```python
from build123d import *

# Parameters (mm, degrees)
SKETCH_1_W               = 50
SKETCH_1_H               = 50
EXTRUDE_1_DEPTH          = 10
SKETCH_2_R               = 1.75
EXTRUDE_2_DEPTH          = 2.25
CUT_EXTRUDE_1_DEPTH      = 71.505318948
CUT_EXTRUDE_1_DEPTH_BACK = 71.505318948
SKETCH_5_R               = 1.75
CUT_EXTRUDE_3_DEPTH      = 71.505318948
CUT_EXTRUDE_3_DEPTH_BACK = 5
SKETCH_6_R               = 3.3
FILLET_1_R               = 10
SKETCH_8_R               = 5.5
CUT_EXTRUDE_5_DEPTH      = 6.5
EXTRUDE_3_DEPTH          = 3
EXTRUDE_4_DEPTH          = 3
FILLET_2_R               = 1


with BuildPart() as part:
    # ｽｹｯﾁ1 → ﾎﾞｽ - 押し出し1 (new body)
    with BuildSketch(Plane(origin=(0, 0, 0), x_dir=(1, 0, 0), z_dir=(0, 1, 0))):
        Rectangle(SKETCH_1_W, SKETCH_1_H)
    extrude(amount=EXTRUDE_1_DEPTH)

    # ｽｹｯﾁ2 → ﾎﾞｽ - 押し出し2 (add, symmetric)
    with BuildSketch(Plane.XY):
        with BuildLine():
            Line((25, 10), (-25, 10))
            Line((-25, 10), (-25, 36))
            ThreePointArc((-25, 36), (0, 61), (25, 36))
            Line((25, 36), (25, 10))
        make_face()
        with Locations((0, 36)):
            Circle(SKETCH_2_R, mode=Mode.SUBTRACT)
    extrude(amount=EXTRUDE_2_DEPTH, both=True)

    # ｽｹｯﾁ5 → ｶｯﾄ - 押し出し1 (cut, two sides: drawn at the far end of the back side and taken through both)
    with BuildSketch(Plane.XY.offset(-CUT_EXTRUDE_1_DEPTH_BACK)):
        with Locations((0, 57)):
            Circle(SKETCH_5_R)
        with Locations((5.435199947, 56.284442352)):
            Circle(SKETCH_5_R)
        with Locations((10.5, 54.186533479)):
            Circle(SKETCH_5_R)
        with Locations((14.849242405, 50.849242405)):
            Circle(SKETCH_5_R)
        with Locations((18.186533479, 46.5)):
            Circle(SKETCH_5_R)
        with Locations((18.186533479, 25.5)):
            Circle(SKETCH_5_R)
        with Locations((14.849242405, 21.150757595)):
            Circle(SKETCH_5_R)
        with Locations((10.5, 17.813466521)):
            Circle(SKETCH_5_R)
        with Locations((5.435199947, 15.715557648)):
            Circle(SKETCH_5_R)
        with Locations((0, 15)):
            Circle(SKETCH_5_R)
        with Locations((-5.435199947, 15.715557648)):
            Circle(SKETCH_5_R)
        with Locations((-10.5, 17.813466521)):
            Circle(SKETCH_5_R)
        with Locations((-14.849242405, 21.150757595)):
            Circle(SKETCH_5_R)
        with Locations((-18.186533479, 25.5)):
            Circle(SKETCH_5_R)
        with Locations((-18.186533479, 46.5)):
            Circle(SKETCH_5_R)
        with Locations((-14.849242405, 50.849242405)):
            Circle(SKETCH_5_R)
        with Locations((-10.5, 54.186533479)):
            Circle(SKETCH_5_R)
        with Locations((-5.435199947, 56.284442352)):
            Circle(SKETCH_5_R)
    extrude(amount=CUT_EXTRUDE_1_DEPTH + CUT_EXTRUDE_1_DEPTH_BACK, mode=Mode.SUBTRACT)

    # ｽｹｯﾁ6 → ｶｯﾄ - 押し出し3 (cut, two sides: drawn at the far end of the back side and taken through both)
    with BuildSketch(Plane(origin=(0, 0, 0), x_dir=(1, 0, 0), z_dir=(0, 1, 0)).offset(-CUT_EXTRUDE_3_DEPTH_BACK)):
        with Locations(Location((-10, -10, 0), (0, 0, 90))):
            Circle(SKETCH_6_R)
        with Locations(Location((10, -10, 0), (0, 0, 90))):
            Circle(SKETCH_6_R)
        with Locations(Location((10, 10, 0), (0, 0, 90))):
            Circle(SKETCH_6_R)
        with Locations(Location((-10, 10, 0), (0, 0, 90))):
            Circle(SKETCH_6_R)
    extrude(amount=CUT_EXTRUDE_3_DEPTH + CUT_EXTRUDE_3_DEPTH_BACK, mode=Mode.SUBTRACT)

    # ﾌｨﾚｯﾄ1
    fillet_1_edges = [part.edges().sort_by_distance(p)[0] for p in [
        (-25, 5, 25),
        (-25, 5, -25),
        (25, 5, -25),
        (25, 5, 25),
    ]]
    fillet(fillet_1_edges, radius=FILLET_1_R)

    # ｽｹｯﾁ8 → ｶｯﾄ - 押し出し5 (cut)
    with BuildSketch(Plane(origin=(0, 10, 0), x_dir=(1, 0, 0), z_dir=(0, 1, 0))):
        with Locations(Location((-10, -10, 0), (0, 0, 270))):
            Circle(SKETCH_8_R)
        with Locations(Location((10, -10, 0), (0, 0, 270))):
            Circle(SKETCH_8_R)
        with Locations(Location((10, 10, 0), (0, 0, 270))):
            Circle(SKETCH_8_R)
        with Locations(Location((-10, 10, 0), (0, 0, 270))):
            Circle(SKETCH_8_R)
    extrude(amount=-CUT_EXTRUDE_5_DEPTH, mode=Mode.SUBTRACT)

    # ｽｹｯﾁ11 → ﾎﾞｽ - 押し出し3 (add)
    with BuildSketch(Plane(origin=(25, 0, 0), x_dir=(0, 0, -1), z_dir=(1, 0, 0))):
        Polygon((-2.25, 19.834192463), (-15, 10), (-2.25, 10), align=None)
        Polygon((15, 10), (2.25, 10), (2.25, 19.834192463), align=None)
    extrude(amount=-EXTRUDE_3_DEPTH)

    # ｽｹｯﾁ12 → ﾎﾞｽ - 押し出し4 (add)
    with BuildSketch(Plane.ZY.offset(25)):
        Polygon((2.25, 19.834192463), (15, 10), (2.25, 10), align=None)
        Polygon((-2.25, 19.834192463), (-15, 10), (-2.25, 10), align=None)
    extrude(amount=-EXTRUDE_4_DEPTH)

    # ﾌｨﾚｯﾄ2
    fillet_2_edges = [part.edges().sort_by_distance(p)[0] for p in [
        (0, 10, 2.25),
        (0, 10, -2.25),
    ]]
    fillet(fillet_2_edges, radius=FILLET_2_R)


solid = part.part
```
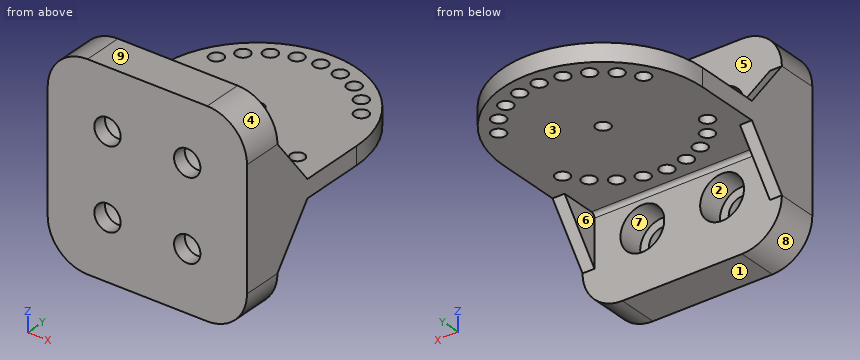
The model under review builds one solid part; all positions refer to its coordinate system, in mm. Face numbers are marked on the shaded views. A direction names the side the tool comes from. Give positions to 0.01 mm unless a question says otherwise; leave off trailing zeros. Write each loop counter-clockwise with the first axis right and the second up, starting at its lowest first coordinate (ties: lowest second). Pieces come first, ordered by that corner, then holes. Notation, with made-up numbers: (-31.5, 62) - (-0.5, 62) arc R16 ccw to (-0.5, 91) - close; hole circle Ø3 at (13, 36). An arc over 180 degrees is marked (long way). Answer in a Markdown table with one row per item. Add a question column.
1. Insertion check: P1, Ø4, axis at x = 10, z = -10, coming from the -Y side (3 decimals); P2, Ø5, axis at x = -18, y = 55, coming from the +Z side; P3, Ø4.5, axis at x = -5.44, y = 56.28, coming from the -Z side; P4, Ø4, axis at x = -18.5, z = -15, coming from the +Y side. Each pin has a flat end and moves straight along its axis. Give the tip position at first contact, or say it passes through.
2. Wall thickness on line 1 along X through (y, z) = (6.75, 10); line 2 along X through (y, z) = (7, -9); line 3 along Y through (x, z) = (3.5, 14): over which ranges is each line inside the solid? List them lowest first. Write a range as [from, to].
3. We need section B-B on y = 25.5. Write out the cut boundary in (x, z).
4. Draft analysis for pull direction Z (two halves, no side actions). For the marked faces 6, 7, 8 and 9, state which applies: +Z half, -Z half, draft (parallel to the pull), parting line (faces both ways), or undercut.
5. Tool access review of the marked faces 1, 2, 3, 4 and 5: name each direction out of +Z, -Z, +X, -X, +Y, -Y from which nothing blocks a thin tool from reaching the whole face with its end or side.
6. We need section A-A on x = 0. Write out the cut boundary in (y, z), then the cut area to 3 significant figures.
7. We need section C-C on x = -10. State how many separate pieces and enclosed holes the cut face has, then the cut area to 3 significant figures.
8. We need section D-D on z = -11. Write out the cut boundary in (x, y), then the cut area to 3 significant figures.
Ans:
| question | item | result |
|---|---|---|
| 1 | P1 | passes through |
| 1 | P2 | stops at z = 2.25 |
| 1 | P3 | stops at z = -2.25 |
| 1 | P4 | stops at y = 10 |
| 2 | line 1 | x = [-25, -15.5], [-4.5, 4.5], [15.5, 25] |
| 2 | line 2 | x = [-25, -15.41], [-4.59, 4.59], [15.41, 25] |
| 2 | line 3 | y = [0, 10] |
| 3 | outline | (-25, -2.25) - (-19.94, -2.25) - (-19.94, 2.25) - (-25, 2.25) - close; (-16.44, -2.25) - (16.44, -2.25) - (16.44, 2.25) - (-16.44, 2.25) - close; (19.94, -2.25) - (25, -2.25) - (25, 2.25) - (19.94, 2.25) - close |
| 4 | face 6 | draft |
| 4 | face 7 | undercut |
| 4 | face 8 | -Z half |
| 4 | face 9 | +Z half |
| 5 | face 1 | -Z, +X, -X, +Y, -Y |
| 5 | face 2 | +Y |
| 5 | face 3 | -Z, +Y |
| 5 | face 4 | +Z, +X, +Y, -Y |
| 5 | face 5 | +Z, +Y |
| 6 | outline | (0, -25) - (10, -25) - (10, -3.25) arc R1 cw to (11, -2.25) - (13.25, -2.25) - (13.25, 2.25) - (11, 2.25) arc R1 cw to (10, 3.25) - (10, 25) - (0, 25) - close; (16.75, -2.25) - (34.25, -2.25) - (34.25, 2.25) - (16.75, 2.25) - close; (37.75, -2.25) - (55.25, -2.25) - (55.25, 2.25) - (37.75, 2.25) - close; (58.75, -2.25) - (61, -2.25) - (61, 2.25) - (58.75, 2.25) - close |
| 6 | area | 683 mm^2 |
| 7 | separate pieces | 5 |
| 7 | enclosed holes | 0 |
| 7 | area | 501 mm^2 |
| 8 | outline | (-25, 0) - (-13.14, 0) - (-13.14, 3.5) - (-15.41, 3.5) - (-15.41, 10) - (-22, 10) - (-22, 13.09) - (-25, 13.09) - close; (-6.86, 0) - (6.86, 0) - (6.86, 3.5) - (4.59, 3.5) - (4.59, 10) - (-4.59, 10) - (-4.59, 3.5) - (-6.86, 3.5) - close; (13.14, 0) - (25, 0) - (25, 13.09) - (22, 13.09) - (22, 10) - (15.41, 10) - (15.41, 3.5) - (13.14, 3.5) - close |
| 8 | area | 334 mm^2 |
